```python
from build123d import *

# Parameters (mm, degrees)
SKETCH1_R           = 2.25
SKETCH1_R_2         = 1.65
BOSS_EXTRUDE1_DEPTH = 1
SKETCH2_R           = 4
SKETCH2_R_2         = 1.65
BOSS_EXTRUDE2_DEPTH = 5
CHAMFER1_SIZE       = 1
CHAMFER1_SIZE_2     = 2.25


with BuildPart() as part:
    # Sketch1 → Boss-Extrude1 (new body)
    with BuildSketch(Plane.XY):
        Circle(SKETCH1_R)
        Circle(SKETCH1_R_2, mode=Mode.SUBTRACT)
    extrude(amount=BOSS_EXTRUDE1_DEPTH)

    # Sketch2 → Boss-Extrude2 (add)
    with BuildSketch(Plane.XY.offset(1)):
        Circle(SKETCH2_R)
        Circle(SKETCH2_R_2, mode=Mode.SUBTRACT)
    extrude(amount=BOSS_EXTRUDE2_DEPTH)

    # Chamfer1
    # the kernel refuses this chamfer: 2.25, 1 mm, written as the material it adds along each edge
    with BuildSketch(Plane(origin=(0, 0, 1), x_dir=(1, 0, 0), z_dir=(0, -1, 0))) as chamfer1_piece_1_section:
        Polygon((2.25, -CHAMFER1_SIZE), (2.25 + CHAMFER1_SIZE_2, 0), (2.25, 0), align=None)
    chamfer1_piece_1 = revolve(axis=Axis((0, 0, 1), (0, 0, 1)), mode=Mode.PRIVATE)
    chamfer1_piece_1 = split(chamfer1_piece_1, bisect_by=Plane(origin=(-3.113599445, 0, 0), z_dir=(0, 0, 1)), keep=Keep.TOP, mode=Mode.PRIVATE)
    chamfer1_piece_1 = chamfer1_piece_1 & Plane(origin=(0, 0, 0.414540138), x_dir=(1, 0, 0), z_dir=(0, 0, -1)) * Cylinder(4, 18, mode=Mode.PRIVATE)
    add(chamfer1_piece_1)


solid = part.part
```
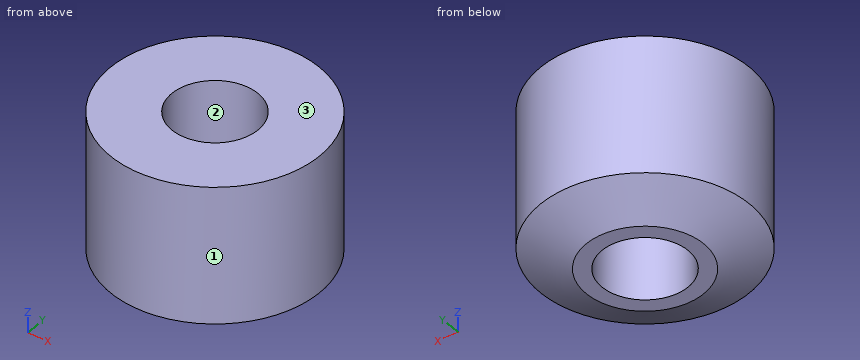
The model under review builds one solid part; all positions refer to its coordinate system, in mm. Face numbers are marked on the shaded views. Round coordinates to 2 decimals unless told otherwise and drop trailing zeros. Loops run counter-clockwise (first coordinate to the right, second up) from the corner with the lowest first, then second, coordinate; pieces in that order, holes last. Notation, with made-up numbers: (30, -31) -> (43, -31) arc R11 ccw to (43, -11) -> close; hole circle Ø8 at (15.5, -25.75). An arc over 180 degrees is marked (long way). Answer as a JSON object with one key per item and string values. Group by question number.
1) We need section A-A on x = 0. Write out the cut boundary in (y, z), then the cut area to 3 significant figures.
2) We need section C-C on z = 3.2. Write out the cut boundary in (x, y), then the cut area to 3 significant figures.
3) For line 1 (Y direction, x = 0, z = 1.3); line 2 (X direction, y = 1.5, z = 4.4); line 3 (Y direction, x = 1.5, z = 0.75), list the stretches that pass through material, from the lowest coordinate up. Write a range as [from, to].
4) Mouldability with a two-part tool opening along X and no side actions: class the marked faces 1, 2 and 3 as released by +X, released by -X, zero draft, split by the parting line, or undercut.
Result set:
{
 "1": {"outline": "(-4, 0.78) -> (-2.25, 0) -> (-1.65, 0) -> (-1.65, 6) -> (-4, 6) -> close; (1.65, 0) -> (2.25, 0) -> (4, 0.78) -> (4, 6) -> (1.65, 6) -> close", "area": "26.8 mm²"},
 "2": {"outline": "circle Ø8 at (0, 0); hole circle Ø3.3 at (0, 0)", "area": "41.7 mm²"},
 "3": {"line 1": "[-4, -1.65], [1.65, 4]", "line 2": "[-3.71, -0.69], [0.69, 3.71]", "line 3": "[-3.64, -0.69], [0.69, 3.64]"},
 "4": {"face 1": "split by the parting line", "face 2": "undercut", "face 3": "zero draft"}
}
